Part model, mm, in its own coordinate system. Face numbers are marked on the shaded views. A direction names the side the tool comes from. Round coordinates to 2 decimals unless told otherwise and drop trailing zeros. Write each loop counter-clockwise with the first axis right and the second up, starting at its lowest first coordinate (ties: lowest second). Pieces come first, ordered by that corner, then holes. Notation, with made-up numbers: M 87,25.5 L 137,25.5 A23 ccw 137,35.5 Z; hole C -2.75,76.25 d2. An arc over 180 degrees is marked long. Answer as a JSON object with one key per item and string values. Group by question number.
1. Drill centre lines: line 1 (X direction, y = -25.8, z = -14.65); line 2 (Y direction, x = 11.2, z = 1.65); line 3 (Y direction, x = 11.2, z = -16.15). Where is each one in solid material? Low to high. Write a range as from..to.
2. Drop flat-ended pins along their axis: pin 1 (2.5 mm diameter, centred on x = 9.9, y = -35.8, fed in from +Z); pin 2 (2.5 mm diameter, centred on y = -0.5, z = 0.5, fed in from -X); pin 3 (4 mm diameter, centred on x = 14, y = 3.5, fed in from -Z). Give the stop position or say it passes through.
3. Band-saw the part on B-B, the plane y = 3.3. Write the cut outline in (x, z), plus the area to 3 significant figures.
4. Band-saw the part on A-A, the plane y = -25.8. Write the cut outline in (x, z).
5. Band-saw the part on C-C, the plane x = 6.5. Write the cut outline in (y, z), plus the area to 3 significant figures.
6. Which spindle directions (+Z, -Z, +X, -X, +Y, -Y) get a long thin tool onto all of the face, cutting with end or side? Do the marked faces 1, 2 and 3. Say none if no direction does.
7. Band-saw the part on D-D, the plane x = 14.25. Write the cut outline in (y, z).
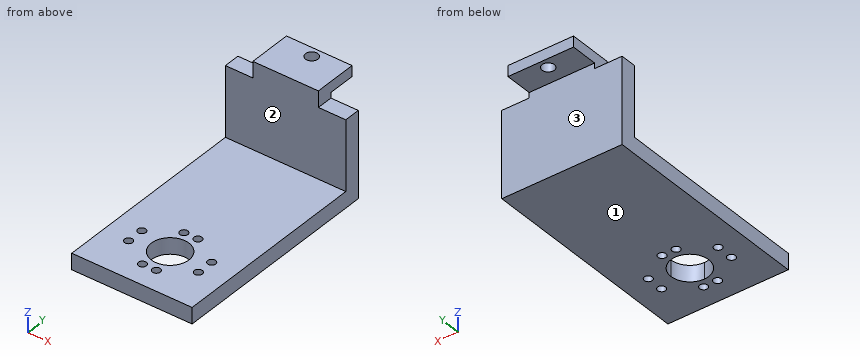
from build123d import *

# Parameters (mm, degrees)
F0_R     = 1.15
F1_DEPTH = 2
F0_W     = 5.1
F0_H     = 3
F2_DEPTH = 17
F3_W     = 22.4
F3_H     = 37
F3_R     = 0.75
F3_H_2   = 3
F4_DEPTH = 3
F5_W     = 5.1
F5_H     = 3
F6_DEPTH = 1


with BuildPart() as f1:
    # F0 (on Top) → F1 (new body)
    with BuildSketch(Plane.XY):
        Polygon((5.1, 0), (11.2, 0), (17.3, 0), (17.3, 5.1), (11.2, 5.1), (5.1, 5.1), align=None)
        with Locations((11.2, 3.3)):
            Circle(F0_R, mode=Mode.SUBTRACT)
        Polygon((17.3, 0), (11.2, 0), (5.1, 0), (5.1, -3), (17.3, -3), align=None)
    extrude(amount=F1_DEPTH)

    # F0 (on Top) → F2 (join)
    with BuildSketch(Plane.XY):
        with Locations((2.55, -1.5)):
            Rectangle(F0_W, F0_H)
        Polygon((17.3, 0), (11.2, 0), (5.1, 0), (5.1, -3), (17.3, -3), align=None)
        with Locations((19.85, -1.5)):
            Rectangle(F0_W, F0_H)
    extrude(amount=-F2_DEPTH)

    # F3 (on face) → F4 (join)
    with BuildSketch(Plane(origin=(0, 0, -17), x_dir=(1, 0, 0), z_dir=(0, 0, -1))):
        with Locations((11.2, 21.5)):
            Rectangle(F3_W, F3_H)
        with Locations((4.6999996006, 29.2)):
            Circle(F3_R, mode=Mode.SUBTRACT)
        with Locations((9.8999996006, 25.8)):
            Circle(F3_R, mode=Mode.SUBTRACT)
        with Locations((4.6999996006, 32.4)):
            Circle(F3_R, mode=Mode.SUBTRACT)
        with BuildLine():
            ThreePointArc((11.1999996006, 34.3), (13.6748733348, 33.2748737342), (14.6999996006, 30.8))
            ThreePointArc((14.6999996006, 30.8), (8.7251258665, 28.3251262658), (11.1999996006, 34.3))
        make_face(mode=Mode.SUBTRACT)
        with Locations((9.8999996006, 35.8)):
            Circle(F3_R, mode=Mode.SUBTRACT)
        with Locations((12.4999996006, 25.8)):
            Circle(F3_R, mode=Mode.SUBTRACT)
        with Locations((17.6999996006, 29.2)):
            Circle(F3_R, mode=Mode.SUBTRACT)
        with Locations((12.4999996006, 35.8)):
            Circle(F3_R, mode=Mode.SUBTRACT)
        with Locations((17.6999996006, 32.4)):
            Circle(F3_R, mode=Mode.SUBTRACT)
        with Locations((11.2, 1.5)):
            Rectangle(F3_W, F3_H_2)
    extrude(amount=-F4_DEPTH)

    # F5 (on face) → F6 (cut)
    with BuildSketch(Plane.XY):
        with Locations((2.55, -1.5)):
            Rectangle(F5_W, F5_H)
        with Locations((19.85, -1.5)):
            Rectangle(F5_W, F5_H)
    extrude(amount=-F6_DEPTH, mode=Mode.SUBTRACT)


solid = f1.part
Worked answers:
{
 "1": {"line 1": "x = 0..9.15, 10.65..11.75, 13.25..22.4", "line 2": "y = -3..2.15, 4.45..5.1", "line 3": "y = -40..-34.3, -27.3..0"},
 "2": {"pin 1": "stops at z = -14", "pin 2": "stops at x = 5.1", "pin 3": "stops at z = 0"},
 "3": {"outline": "M 5.1,0 L 10.05,0 L 10.05,2 L 5.1,2 Z; M 12.35,0 L 17.3,0 L 17.3,2 L 12.35,2 Z", "area": "19.8 mm^2"},
 "4": {"outline": "M 0,-17 L 9.15,-17 L 9.15,-14 L 0,-14 Z; M 10.65,-17 L 11.75,-17 L 11.75,-14 L 10.65,-14 Z; M 13.25,-17 L 22.4,-17 L 22.4,-14 L 13.25,-14 Z"},
 "5": {"outline": "M -40,-17 L 0,-17 L 0,0 L 5.1,0 L 5.1,2 L -3,2 L -3,-14 L -40,-14 Z", "area": "178 mm^2"},
 "6": {"face 1": "-Z, +X, -X, +Y, -Y", "face 2": "+Z, +X, -X, -Y", "face 3": "-Z, +X, -X, +Y"},
 "7": {"outline": "M -40,-17 L -32.52,-17 L -32.52,-14 L -40,-14 Z; M -29.08,-17 L 0,-17 L 0,0 L 5.1,0 L 5.1,2 L -3,2 L -3,-14 L -29.08,-14 Z"}
}
